Design review of the part built by this model. Coordinates are the model's own, in mm. A direction names the side the tool comes from. Round coordinates to 2 decimals unless told otherwise and drop trailing zeros. Loops run counter-clockwise (first coordinate to the right, second up) from the corner with the lowest first, then second, coordinate; pieces in that order, holes last. Notation, with made-up numbers: (75.5, 49) - (99.5, 49) arc R27 cw to (99.5, 70) - close; hole circle Ø8 at (15.25, 12.25). An arc over 180 degrees is marked (long way). Return JSON: item names as keys, results as strings. Group by question number.
from build123d import *

# Parameters (mm, degrees)
STOCK_MOUNT_START                              = 19
STOCK_MOUNT_FOR_MOTOR_IN_THE_PLATYFO_2_W       = 50
STOCK_MOUNT_FOR_MOTOR_IN_THE_PLATYFO_2_H       = 57
STOCK_MOUNT_FOR_MOTOR_IN_THE_PLATYFO_2_R       = 1.5
STOCK_MOUNT_FOR_MOTOR_IN_THE_PLATYFO_2_R_2     = 6
STOCK_MOUNT_FOR_MOTOR_IN_THE_PLATYFORM_M_DEPTH = 15
SKETCH2_W                                      = 15
SKETCH2_H                                      = 57
BOSS_EXTRUDE1_DEPTH                            = 19.12
SKETCH3_W                                      = 15
SKETCH3_H                                      = 57
BOSS_EXTRUDE2_DEPTH                            = 19.12
SKETCH4_W                                      = 15
SKETCH4_H                                      = 15
BOSS_EXTRUDE3_DEPTH                            = 20
SKETCH10_W                                     = 15
SKETCH10_H                                     = 65
BOSS_EXTRUDE6_DEPTH                            = 40
SKETCH11_R                                     = 6
SKETCH11_R_2                                   = 2.5
CUT_EXTRUDE2_DEPTH                             = 132.238616268


# Read off the part's stored shape, not the designer's step: Stock-mount for motor in the platyform mechanism-1
with BuildPart() as part:
    # Stock-mount for motor in the platyfo 2 → Stock-mount for motor in the platyform mechanism-1 (new body)
    with BuildSketch(Plane.YZ.offset(STOCK_MOUNT_START)):
        with Locations((-35, 4.5)):
            Rectangle(STOCK_MOUNT_FOR_MOTOR_IN_THE_PLATYFO_2_W, STOCK_MOUNT_FOR_MOTOR_IN_THE_PLATYFO_2_H)
        with Locations((-42.6325, -8.719877789)):
            Circle(STOCK_MOUNT_FOR_MOTOR_IN_THE_PLATYFO_2_R, mode=Mode.SUBTRACT)
        with Locations((-27.3675, -8.719877789)):
            Circle(STOCK_MOUNT_FOR_MOTOR_IN_THE_PLATYFO_2_R, mode=Mode.SUBTRACT)
        with Locations((-50.265, 4.5)):
            Circle(STOCK_MOUNT_FOR_MOTOR_IN_THE_PLATYFO_2_R, mode=Mode.SUBTRACT)
        with Locations((-42.6325, 17.719877789)):
            Circle(STOCK_MOUNT_FOR_MOTOR_IN_THE_PLATYFO_2_R, mode=Mode.SUBTRACT)
        with Locations((-35, 12.5)):
            Circle(STOCK_MOUNT_FOR_MOTOR_IN_THE_PLATYFO_2_R_2, mode=Mode.SUBTRACT)
        with Locations((-27.3675, 17.719877789)):
            Circle(STOCK_MOUNT_FOR_MOTOR_IN_THE_PLATYFO_2_R, mode=Mode.SUBTRACT)
        with Locations((-19.735, 4.5)):
            Circle(STOCK_MOUNT_FOR_MOTOR_IN_THE_PLATYFO_2_R, mode=Mode.SUBTRACT)
    extrude(amount=STOCK_MOUNT_FOR_MOTOR_IN_THE_PLATYFORM_M_DEPTH)

    # Sketch2 → Boss-Extrude1 (add)
    with BuildSketch(Plane.XZ.offset(60)):
        with Locations((26.5, 4.5)):
            Rectangle(SKETCH2_W, SKETCH2_H)
    extrude(amount=BOSS_EXTRUDE1_DEPTH)

    # Sketch3 → Boss-Extrude2 (add)
    with BuildSketch(Plane(origin=(0, -10, 0), x_dir=(1, 0, 0), z_dir=(0, 1, 0))):
        with Locations((26.5, -4.5)):
            Rectangle(SKETCH3_W, SKETCH3_H)
    extrude(amount=BOSS_EXTRUDE2_DEPTH)

    # Sketch4 → Boss-Extrude3 (add)
    with BuildSketch(Plane.XY.offset(33)):
        with Locations((26.5, 1.62)):
            Rectangle(SKETCH4_W, SKETCH4_H)
        with Locations((26.5, -71.62)):
            Rectangle(SKETCH4_W, SKETCH4_H)
    extrude(amount=BOSS_EXTRUDE3_DEPTH)

    # Sketch10 → Boss-Extrude6 (add)
    with BuildSketch(Plane(origin=(0, -79.12, 0), x_dir=(-1, 0, 0), z_dir=(0, -1, 0))):
        with Locations((-26.5, -20.5)):
            Rectangle(SKETCH10_W, SKETCH10_H)
    boss_extrude6 = extrude(amount=BOSS_EXTRUDE6_DEPTH)

    # Mirror1: Boss-Extrude6 across plane
    add(boss_extrude6.mirror(Plane.ZX.offset(-35)))

    # Sketch11 → Cut-Extrude2 (cut, through all)
    with BuildSketch(Plane.ZY.offset(-19)):
        with Locations(Location((20.5, -102.12, 0), (0, 0, 270))):
            Circle(SKETCH11_R)
        with Locations(Location((2.5, -102.12, 0), (0, 0, 270))):
            Circle(SKETCH11_R_2)
        with Locations(Location((38.5, -102.12, 0), (0, 0, 90))):
            Circle(SKETCH11_R_2)
        with Locations(Location((38.5, 32.12, 0), (0, 0, 270))):
            Circle(SKETCH11_R_2)
        with Locations(Location((20.5, 32.12, 0), (0, 0, 90))):
            Circle(SKETCH11_R)
        with Locations(Location((2.5, 32.12, 0), (0, 0, 90))):
            Circle(SKETCH11_R_2)
    extrude(amount=-CUT_EXTRUDE2_DEPTH, mode=Mode.SUBTRACT)


solid = part.part
Q1. Add section A-A, the plane z = 12.5. State the section outline as (x, y) points.
Q2. Draft analysis for pull direction Y (two halves, no side actions). For faces 1 (the flat face through (26, -79.12, -18)), 2 (the flat face through (27, 21, 53)), 3 (the cylindrical face through (26.4, 29.81, 37.54)), state which applies: pulls with the +Y half, pulls with the -Y half, needs draft (parallel to the pull), parting line crosses it, or undercut.
Q3. Add section B-B, the plane y = -35. State the section outline as (x, z) points, plus the area to 3 significant figures.
Q4. Add section D-D, the plane y = 32.12. State the section outline as (x, z) points, plus the area to 3 significant figures.
Q5. Tool access review of faces 4 (the flat face through (27, -91, 53)), 5 (the flat face through (27, -99, -12)), 6 (the flat face through (27, 29, -12)), 7 (the flat face through (26, -64.12, 43)): name each direction out of +Z, -Z, +X, -X, +Y, -Y from which nothing blocks a thin tool from reaching the whole face with its end or side.
Q6. Add section C-C, the plane z = 38.5. State the section outline as (x, y) points, plus the area to 3 significant figures.
Q7. For line 1 (Y direction, x = 32.5, z = 47.5); line 2 (Y direction, x = 25, z = 19); line 3 (Y direction, x = 31.5, z = -9.5), list the stretches that pass through material, from the lowest coordinate up.
Q8. Insertion check: pin 1 Ø3.5 at (x, z) = (25.5, -16.5) entering from +Y. The pin has a flat end and moves straight along its axis. Give the tip position at first contact, or say it passes through.
Evaluation:
{
 "1": {"outline": "(19, -119.12) - (34, -119.12) - (34, -41) - (19, -41) - close; (19, -29) - (34, -29) - (34, 49.12) - (19, 49.12) - close"},
 "2": {"face 1": "pulls with the -Y half", "face 2": "needs draft", "face 3": "undercut"},
 "3": {"outline": "(19, -24) - (34, -24) - (34, 6.5) - (19, 6.5) - close; (19, 18.5) - (34, 18.5) - (34, 33) - (19, 33) - close", "area": "675 mm²"},
 "4": {"outline": "(19, -12) - (34, -12) - (34, 0) - (19, 0) - close; (19, 5) - (34, 5) - (34, 14.5) - (19, 14.5) - close; (19, 26.5) - (34, 26.5) - (34, 36) - (19, 36) - close; (19, 41) - (34, 41) - (34, 53) - (19, 53) - close", "area": "645 mm²"},
 "5": {"face 4": "+Z, +X, -X, +Y, -Y", "face 5": "-Z, +X, -X, -Y", "face 6": "-Z, +X, -X, +Y", "face 7": "+Z, +X, -X"},
 "6": {"outline": "(19, -119.12) - (34, -119.12) - (34, -104.62) - (19, -104.62) - close; (19, -99.62) - (34, -99.62) - (34, -64.12) - (19, -64.12) - close; (19, -5.88) - (34, -5.88) - (34, 29.62) - (19, 29.62) - close; (19, 34.62) - (34, 34.62) - (34, 49.12) - (19, 49.12) - close", "area": "1,500 mm²"},
 "7": {"line 1": "-119.12 to -64.12, -5.88 to 49.12", "line 2": "-119.12 to -107.93, -96.31 to -43.41, -41.85 to -28.15, -26.59 to 26.31, 37.93 to 49.12", "line 3": "-119.12 to -43.91, -41.35 to -28.65, -26.09 to 49.12"},
 "8": {"pin 1": "y = 9.12"}
}
